Build history of the part. All positions in model axes, mm. Give positions to 0.01 mm unless a question says otherwise; leave off trailing zeros. Write each loop counter-clockwise with the first axis right and the second up, starting at its lowest first coordinate (ties: lowest second). Pieces come first, ordered by that corner, then holes. Notation, with made-up numbers: M -19.75,-28.5 L 12.25,-28.5 A34 cw 12.25,3.5 Z; hole C 65,49.25 d1. An arc over 180 degrees is marked long. Return JSON: item names as keys, results as strings. Group by question number.
Q1. Flat gauge pin, fed straight in: pin 1 Ø1.5 at (y, z) = (2, 0.5) entering from +X. Where does the tip first touch, or does it go through?
Q2. Band-saw the part on D-D, the plane z = 1.5. Give the cut face in (x, y).
Q3. Band-saw the part on A-A, the plane x = 0. Give the cut face in (y, z).
Q4. Band-saw the part on C-C, the plane z = 2.6. Give the cut face in (x, y), then the cut area to 3 significant figures.
Q5. Wall check: probe 1 along Y at (x, z) = (0, 1.8); probe 2 along Y at (x, z) = (1.1, 2.35); probe 3 along X at (y, z) = (1.6, 1.2). Give the ranges that are in metal, low to high.
Q6. Pull direction Y, two halves, no side cores. Call faces 1 (the cylindrical face through (-3, 0, 1)), 2 (the flat face through (1, -2, 0)), 3 (the cylindrical face through (-1.5, 0.07, 1.49)): +Y half, -Y half, draft (parallel to the pull), parting line (faces both ways), or undercut.
from build123d import *

# Parameters (mm, degrees)
SCHIZZO1_R                   = 3
SCHIZZO1_R_2                 = 1.5
ESTRUSIONE_ESTRUSIONE1_DEPTH = 3
SMUSSO1_SIZE                 = 0.5
CHAMFER1_SIZE                = 0.5


with BuildPart() as part:
    # Schizzo1 → Estrusione-Estrusione1 (new body)
    with BuildSketch(Plane.XY):
        Circle(SCHIZZO1_R)
        Circle(SCHIZZO1_R_2, mode=Mode.SUBTRACT)
    extrude(amount=ESTRUSIONE_ESTRUSIONE1_DEPTH)

    # Smusso1
    smusso1_edges = [part.edges().sort_by_distance(p)[0] for p in [
        (-1.5, 0, 3),
    ]]
    chamfer(smusso1_edges, length=SMUSSO1_SIZE)

    # Chamfer1
    chamfer1_edges = [part.edges().sort_by_distance(p)[0] for p in [
        (-1.5, 0, 0),
    ]]
    chamfer(chamfer1_edges, length=CHAMFER1_SIZE)


solid = part.part
From the geometry:
{
 "1": {"pin 1": "stops at x = 2.73"},
 "2": {"outline": "C 0,0 d6; hole C 0,0 d3"},
 "3": {"outline": "M -3,0 L -2,0 L -1.5,0.5 L -1.5,2.5 L -2,3 L -3,3 Z; M 1.5,0.5 L 2,0 L 3,0 L 3,3 L 2,3 L 1.5,2.5 Z"},
 "4": {"outline": "C 0,0 d6; hole C 0,0 d3.2", "area": "20.2 mm^2"},
 "5": {"probe 1": "y = -3 to -1.5, 1.5 to 3", "probe 2": "y = -2.79 to -1.02, 1.02 to 2.79", "probe 3": "x = -2.54 to 2.54"},
 "6": {"face 1": "parting line", "face 2": "draft", "face 3": "undercut"}
}
